For this review, take the finished solid that the model builds, in its own axes (mm). Give positions to 0.01 mm unless a question says otherwise; leave off trailing zeros. Loops run counter-clockwise (first coordinate to the right, second up) from the corner with the lowest first, then second, coordinate; pieces in that order, holes last. Notation, with made-up numbers: (30.25, 70) - (49.25, 70) arc R11 cw to (49.25, 76) - close; hole circle Ø5 at (37.5, 24.25). An arc over 180 degrees is marked (long way). Answer as CSV lines item,"result".
Autodesk Inventor part; units mm, degrees
ref_plane "YZ Plane" through (0, 0, 0) normal (1, 0, 0) x (0, 1, 0)
ref_plane "XZ Plane" through (0, 0, 0) normal (0, 1, 0) x (-1, 0, 0)
ref_plane "XY Plane" through (0, 0, 0) normal (0, 0, 1) x (1, 0, 0)
sketch "Sketch1" plane through (0, 0, 0) normal (0, 0, 1) x (1, 0, 0)
  circle A0 centre (0, 0) radius 3.0625
  circle A1 centre (0, 0) radius 5.0625
  dimension "d0" = 6.125
  dimension "d1" = 2
extrude "Extrusion1" add sketch "Sketch1" along normal blind 2.5
sketch "Sketch2" plane through (0, 0, 0) normal (0, 0, -1) x (-1, 0, 0)
  circle A0 centre (0, 0) radius 5.0625
  circle A1 centre (0, 0) radius 4.0625
  circle A2 centre (0, 0) radius 8.0625
  dimension "d4" = 8.125
  dimension "d5" = 4
extrude "Extrusion2" add sketch "Sketch2" along normal blind 2 contours A0 | A2
sketch "Sketch3" plane through (0, 0, 0) normal (0, 0, 1) x (1, 0, 0)
  circle A0 centre (0, 0) radius 8.0625
  circle A1 centre (0, 0) radius 5.0625
extrude "Extrusion3" add sketch "Sketch3" along normal up to surface (2.5 mm away)
chamfer "Chamfer1" distance 0.25 angle 45 2 edges at (4.0625, 0, 0) (-3.0625, 0, 0)
properties part number "ArmBaseEncoderAlignmentFlange"
1) Insertion check: P1, Ø1.5, axis at x = -2.5, y = 3, coming from the -Z side; P2, Ø5, axis at x = 0, y = 0, coming from the -Z side; P3, Ø1.5, axis at y = 2, z = -0.5, coming from the -X side (3 decimals); P4, Ø1.5, axis at x = 4.5, z = 0.5, coming from the -Y side. Each pin has a flat end and moves straight along its axis. Give the tip position at first contact, or say it passes through.
From the geometry:
P1,"stops at z = -2"
P2,"passes through"
P3,"stops at x = -7.965"
P4,"stops at y = -7.14"
2) Wall thickness on line 1 (Y direction, x = 0, z = 1.8); line 2 (Y direction, x = 0, z = -0.95); line 3 (X direction, y = 1.25, z = -1.2): over which ranges is each line inside the solid? List them lowest first. Write a range as from..to.
From the geometry:
line 1,"y = -8.06..-3.06, 3.06..8.06"
line 2,"y = -8.06..-4.06, 4.06..8.06"
line 3,"x = -7.97..-3.87, 3.87..7.97"
3) Consider section A-A on y = 0. Write out the cut boundary in (x, z).
From the geometry:
outline,"(-8.06, -2) - (-4.06, -2) - (-4.06, -0.25) - (-3.81, 0) - (-3.31, 0) - (-3.06, 0.25) - (-3.06, 2.5) - (-8.06, 2.5) - close; (3.06, 0.25) - (3.31, 0) - (3.81, 0) - (4.06, -0.25) - (4.06, -2) - (8.06, -2) - (8.06, 2.5) - (3.06, 2.5) - close"
4) Consider section C-C on z = -0.9. Write out the cut boundary in (x, y) (1 decimal).
From the geometry:
outline,"circle Ø16.1 at (0, 0); hole circle Ø8.1 at (0, 0)"
5) Draft analysis for pull direction X (two halves, no side actions). For faces 1 (the cylindrical face through (-3.875, -1.22, -1.113)), 2 (the flat face through (4, 2, -2)), 3 (the flat face through (-3, 2, 0)), state which applies: pulls with the +X half, pulls with the -X half, needs draft (parallel to the pull), parting line crosses it, or undercut.
From the geometry:
face 1,"undercut"
face 2,"needs draft"
face 3,"undercut"
6) Consider section D-D on y = 5.75. Write out the cut boundary in (x, z).
From the geometry:
outline,"(-5.65, -2) - (5.65, -2) - (5.65, 2.5) - (-5.65, 2.5) - close"
